Geometry check sheet. Reference: drawing and pictorial views, mm from the part's lowest x, y, z. A direction names the side the tool comes from. Round coordinates to 2 decimals unless told otherwise and drop trailing zeros. Loops run counter-clockwise (first coordinate to the right, second up) from the corner with the lowest first, then second, coordinate; pieces in that order, holes last. Notation, with made-up numbers: (-4.75, 26) -> (53.25, 26) arc R13 cw to (53.25, 45) -> close; hole circle Ø9 at (3, -13.5). An arc over 180 degrees is marked (long way). Use one line per item in the form item = value.
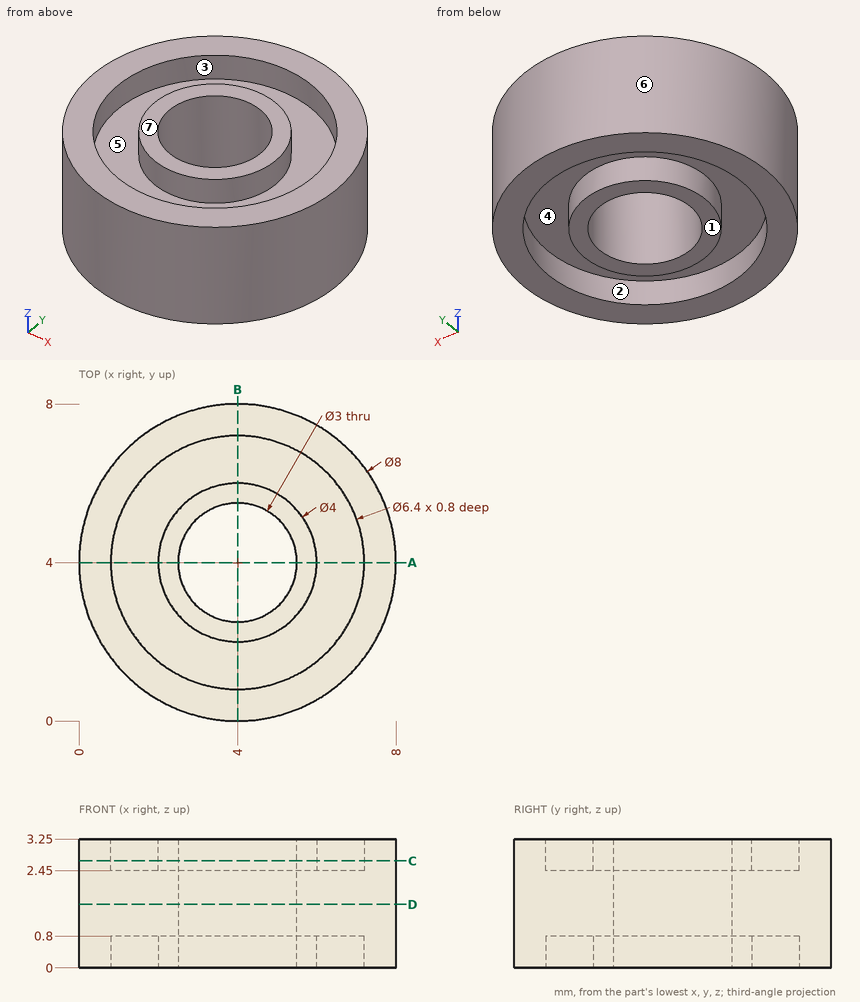
1. Material ranges on line 1 along Y through (x, z) = (4, 0.3); line 2 along X through (y, z) = (4.5, 0.65); line 3 along Y through (x, z) = (6.5, 0.5), recorded low to high.
Return value:
line_1 = 0 to 0.8, 2 to 2.5, 5.5 to 6, 7.2 to 8
line_2 = 0.03 to 0.84, 2.06 to 2.59, 5.41 to 5.94, 7.16 to 7.97
line_3 = 0.88 to 2, 6 to 7.12
2. Tool access check on the marked faces 1, 2 and 3. Record the directions out of +Z, -Z, +X, -X, +Y, -Y that give a thin tool (end or side, any length) a straight path to the whole face; none if there is none.
Return value:
face_1 = -Z, +X, -X, +Y, -Y
face_2 = -Z
face_3 = +Z
3. Mould release check, pull along X, two halves, no side actions. Record for the marked faces 4, 5, 6 and 7: released by +X, released by -X, zero draft, split by the parting line, or undercut.
Return value:
face_4 = undercut
face_5 = undercut
face_6 = split by the parting line
face_7 = zero draft
4. Section check C-C (z = 2.7). Record the boundary of the cut face in (x, y).
Return value:
outline = circle Ø8 at (4, 4); circle Ø4 at (4, 4); hole circle Ø6.4 at (4, 4); hole circle Ø3 at (4, 4)
5. Section check A-A (y = 4). Record the boundary of the cut face in (x, z), then the cut area to 3 significant figures.
Return value:
outline = (0, 0) -> (0.8, 0) -> (0.8, 0.8) -> (2, 0.8) -> (2, 0) -> (2.5, 0) -> (2.5, 3.25) -> (2, 3.25) -> (2, 2.45) -> (0.8, 2.45) -> (0.8, 3.25) -> (0, 3.25) -> close; (5.5, 0) -> (6, 0) -> (6, 0.8) -> (7.2, 0.8) -> (7.2, 0) -> (8, 0) -> (8, 3.25) -> (7.2, 3.25) -> (7.2, 2.45) -> (6, 2.45) -> (6, 3.25) -> (5.5, 3.25) -> close
area = 12.4 mm2
6. Section check D-D (z = 1.6). Record the boundary of the cut face in (x, y), then the cut area to 3 significant figures.
Return value:
outline = circle Ø8 at (4, 4); hole circle Ø3 at (4, 4)
area = 43.2 mm2
7. Gauge pin test, flat ends, axial feed: pin 1 (1.5 mm diameter, centred on y = 2, z = 0.5, fed in from +X); pin 2 (1.8 mm diameter, centred on x = 4, y = 4, fed in from +Z). Record the tip position at first contact, or that the pin passes through.
Return value:
pin_1 = 7.8
pin_2 = through
